Here's how the part is built. I have some questions about the finished solid (model axes, mm). Give positions to 0.01 mm unless a question says otherwise; leave off trailing zeros. Order: outer loops, then holes, each group sorted by start corner. A loop starts at its lowest first (then second) coordinate and runs counter-clockwise, first axis right, second up. Notation, with made-up numbers: M 7,-18 L 23,-18 A18 cw 23,-4 Z; hole C 32.5,72 d9. An arc over 180 degrees is marked long. Use one line per item in the form item = value.
Autodesk Inventor part; units mm, degrees
ref_plane "YZ Plane" through (0, 0, 0) normal (1, 0, 0) x (0, 1, 0)
ref_plane "XZ Plane" through (0, 0, 0) normal (0, 1, 0) x (-1, 0, 0)
ref_plane "XY Plane" through (0, 0, 0) normal (0, 0, 1) x (1, 0, 0)
sketch "Sketch1" plane through (0, 0, 0) normal (0, 0, 1) x (1, 0, 0)
  line L0 (0, 0) -> (-101.6, 0)
  line L1 (-101.6, 0) -> (-101.6, 50.8)
  line L2 (-101.6, 50.8) -> (0, 50.8)
  line L3 (0, 50.8) -> (0, 0)
  circle A0 centre (-82.55, 25.4) radius 2.5527
  circle A1 centre (-19.05, 25.4) radius 2.5527
  dimension "holewidth" = 5.1054
  dimension "d1" = 5.1054
  dimension "d2" = 50.8
  dimension "d3" = 101.6
  dimension "d6" = 63.5
  dimension "d7" = 19.05
  dimension "d8" = 25.4
  dimension "d9" = 19.05
extrude "Plate1" add sketch "Sketch1" along normal blind 3.048
equation "\"d1\" = holewidth"
equation "\"BendRadius\" = Thickness"
equation "\"BendReliefWidth\" = Thickness"
equation "\"BendReliefDepth\" = 0.5 * Thickness"
equation "\"CornerReliefSize\" = 4 * Thickness"
equation "\"MinimumRemnant\" = 2 * Thickness"
equation "\"TransitionRadius\" = BendRadius"
equation "\"JacobiRadiusSize\" = BendRadius"
equation "\"GapSize\" = Thickness"
equation "\"d10\" = BendRadius"
properties part number "Nano Mounting Plate"
Q1. I need wall thicknesses on L1, parallel to Y at x = -82.55, z = 1.3. Which ranges of the line are inside material? Lowest first, please.
Found:
L1 = 0 to 22.85, 27.95 to 50.8
Q2. Thinking about a two-plate mould opening in X: for faces 1 (the face through (-16.7, 26.4, 1.5)), 2 (the face through (-52, 50.8, 2)), 3 (the face through (0, 26, 2)), 4 (the face through (-85.1, 25.3, 1.5)), which applies, +X half, -X half, draft (parallel to the pull), parting line (faces both ways), or undercut?
Found:
face_1 = undercut
face_2 = draft
face_3 = +X half
face_4 = undercut
Q3. I want a section at A-A on y = 25.4. Write out the boundary of the cut face in (x, z), then the cut area to 3 significant figures.
Found:
outline = M -101.6,0 L -85.1,0 L -85.1,3.05 L -101.6,3.05 Z; M -80,0 L -21.6,0 L -21.6,3.05 L -80,3.05 Z; M -16.5,0 L 0,0 L 0,3.05 L -16.5,3.05 Z
area = 279 mm²
Q4. I want a section at B-B on x = -19.05. Write out the boundary of the cut face in (y, z).
Found:
outline = M 0,0 L 22.85,0 L 22.85,3.05 L 0,3.05 Z; M 27.95,0 L 50.8,0 L 50.8,3.05 L 27.95,3.05 Z
